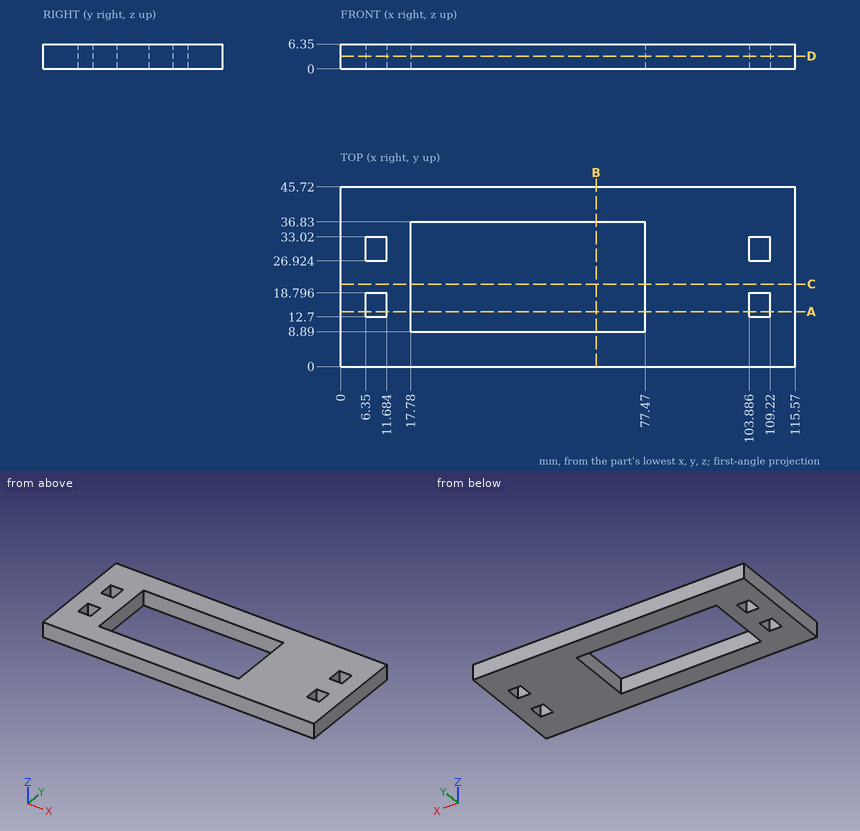
Design review of the part shown in the three views and the two pictorial views. Dimensions are in mm from the part's minimum x, y and z. Round coordinates to 2 decimals unless told otherwise and drop trailing zeros. Order: outer loops, then holes, each group sorted by start corner. A loop starts at its lowest first (then second) coordinate and runs counter-clockwise, first axis right, second up.
Q1. We need section D-D, the plane z = 3.25. Give the boundary of the cut face in (x, y), plus the area to 3 significant figures.
Findings below:
outline: (0, 0) - (115.57, 0) - (115.57, 45.72) - (0, 45.72) - close; hole (6.35, 12.7) - (11.68, 12.7) - (11.68, 18.8) - (6.35, 18.8) - close; hole (6.35, 26.92) - (11.68, 26.92) - (11.68, 33.02) - (6.35, 33.02) - close; hole (17.78, 8.89) - (77.47, 8.89) - (77.47, 36.83) - (17.78, 36.83) - close; hole (103.89, 12.7) - (109.22, 12.7) - (109.22, 18.8) - (103.89, 18.8) - close; hole (103.89, 26.92) - (109.22, 26.92) - (109.22, 33.02) - (103.89, 33.02) - close
area: 3,490 mm2
Q2. Insertion check: P1, Ø3, axis at x = 59, z = 3, coming from the -Y side. The pin has a flat end and moves straight along its axis. Give the tip position at first contact, or say it passes through.
Findings below:
P1: stops at y = 0
Q3. We need section A-A, the plane y = 14. Give the boundary of the cut face in (x, z), plus the area to 3 significant figures.
Findings below:
outline: (0, 0) - (6.35, 0) - (6.35, 6.35) - (0, 6.35) - close; (11.68, 0) - (17.78, 0) - (17.78, 6.35) - (11.68, 6.35) - close; (77.47, 0) - (103.89, 0) - (103.89, 6.35) - (77.47, 6.35) - close; (109.22, 0) - (115.57, 0) - (115.57, 6.35) - (109.22, 6.35) - close
area: 287 mm2
Q4. We need section C-C, the plane y = 21. Give the boundary of the cut face in (x, z), plus the area to 3 significant figures.
Findings below:
outline: (0, 0) - (17.78, 0) - (17.78, 6.35) - (0, 6.35) - close; (77.47, 0) - (115.57, 0) - (115.57, 6.35) - (77.47, 6.35) - close
area: 355 mm2
Q5. We need section B-B, the plane x = 65. Give the boundary of the cut face in (y, z).
Findings below:
outline: (0, 0) - (8.89, 0) - (8.89, 6.35) - (0, 6.35) - close; (36.83, 0) - (45.72, 0) - (45.72, 6.35) - (36.83, 6.35) - close
Q6. Wall thickness on line 1 (X direction, y = 13, z = 3.75); line 2 (Y direction, x = 106, z = 4.25); line 3 (Y direction, x = 30, z = 1.25): over which ranges is each line inside the solid? List them lowest first.
Findings below:
line 1: x = 0 to 6.35, 11.68 to 17.78, 77.47 to 103.89, 109.22 to 115.57
line 2: y = 0 to 12.7, 18.8 to 26.92, 33.02 to 45.72
line 3: y = 0 to 8.89, 36.83 to 45.72
